Solid Edge part; units mm, degrees
sketch "Sketch1" plane through (0, 0, 0) normal (0, -1, 0) x (1, 0, 0)
  line L0 (23.3391, 70.9) -> (23.3391, 66.3391)
  line L1 (23.3391, 66.3391) -> (21, 64)
  line L2 (21, 64) -> (21, 44)
  line L3 (35, 30) -> (21, 44)
  line L4 (35, 0) -> (35, 30)
  line L5 (30, 0) -> (35, 0)
  line L6 (30, 27.9289) -> (30, 0)
  line L7 (16, 41.9289) -> (30, 27.9289)
  line L8 (16, 70.9) -> (16, 41.9289)
  line L9 (16, 70.9) -> (23.3391, 70.9)
revolve "RevolvedProtrusion1" add sketch "Sketch1" angle 360 about axis through (0, 0, 0) along (0, 0, 1)
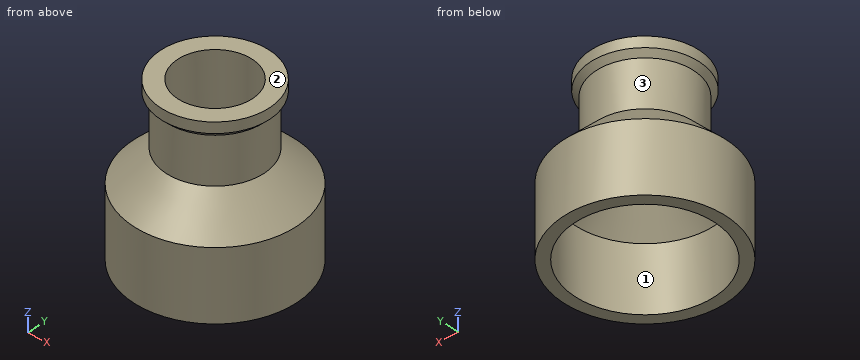
Part model, mm, in its own coordinate system. Face numbers are marked on the shaded views. Round coordinates to 2 decimals unless told otherwise and drop trailing zeros. Loops run counter-clockwise (first coordinate to the right, second up) from the corner with the lowest first, then second, coordinate; pieces in that order, holes last. Notation, with made-up numbers: (-20, -27.75) -> (3, -27.75) arc R33 ccw to (3, 8.25) -> close; hole circle Ø4 at (-29.75, 31.5). An arc over 180 degrees is marked (long way). Use a Markdown table: item, result.
1) Cut at A-A, the plane y = 0. List the corners of the cut face in (x, z), and give its area (3 significant figures).
The answers:
| item | result |
|---|---|
| outline | (-35, 0) -> (-30, 0) -> (-30, 27.93) -> (-16, 41.93) -> (-16, 70.9) -> (-23.34, 70.9) -> (-23.34, 66.34) -> (-21, 64) -> (-21, 44) -> (-35, 30) -> close; (16, 41.93) -> (30, 27.93) -> (30, 0) -> (35, 0) -> (35, 30) -> (21, 44) -> (21, 64) -> (23.34, 66.34) -> (23.34, 70.9) -> (16, 70.9) -> close |
| area | 794 mm2 |
2) Pull direction Y, two halves, no side cores. Call the marked faces 1, 2 and 3: pulls with the +Y half, pulls with the -Y half, needs draft (parallel to the pull), parting line crosses it, or undercut.
The answers:
| item | result |
|---|---|
| face 1 | undercut |
| face 2 | needs draft |
| face 3 | parting line crosses it |
3) Drop flat-ended pins along their axis: pin 1 Ø6 at (y, z) = (-7.5, 40) entering from +X; pin 2 Ø1.5 at (x, z) = (-1, 17.5) entering from +Y; pin 3 Ø4 at (x, y) = (-23, -18) entering from +Z; pin 4 Ø8 at (x, y) = (27, -2) entering from -Z. Give the stop position or say it passes through.
The answers:
| item | result |
|---|---|
| pin 1 | stops at x = 27.08 |
| pin 2 | stops at y = 35 |
| pin 3 | stops at z = 37.79 |
| pin 4 | stops at z = 0 |
4) Cut at C-C, the plane z = 58.5. List the corners of the cut face in (x, y), and give its area (3 significant figures).
The answers:
| item | result |
|---|---|
| outline | circle Ø42 at (0, 0); hole circle Ø32 at (0, 0) |
| area | 581 mm2 |
5) Cut at D-D, the plane z = 26. List the corners of the cut face in (x, y).
The answers:
| item | result |
|---|---|
| outline | circle Ø70 at (0, 0); hole circle Ø60 at (0, 0) |
6) Probe line 1 (Y direction, x = 0, z = 13); line 2 (Y direction, x = 0, z = 60); line 3 (X direction, y = 21, z = 3.5). List the from-to ranges inside material, lowest first. Write a range as [from, to].
The answers:
| item | result |
|---|---|
| line 1 | y = [-35, -30], [30, 35] |
| line 2 | y = [-21, -16], [16, 21] |
| line 3 | x = [-28, -21.42], [21.42, 28] |
